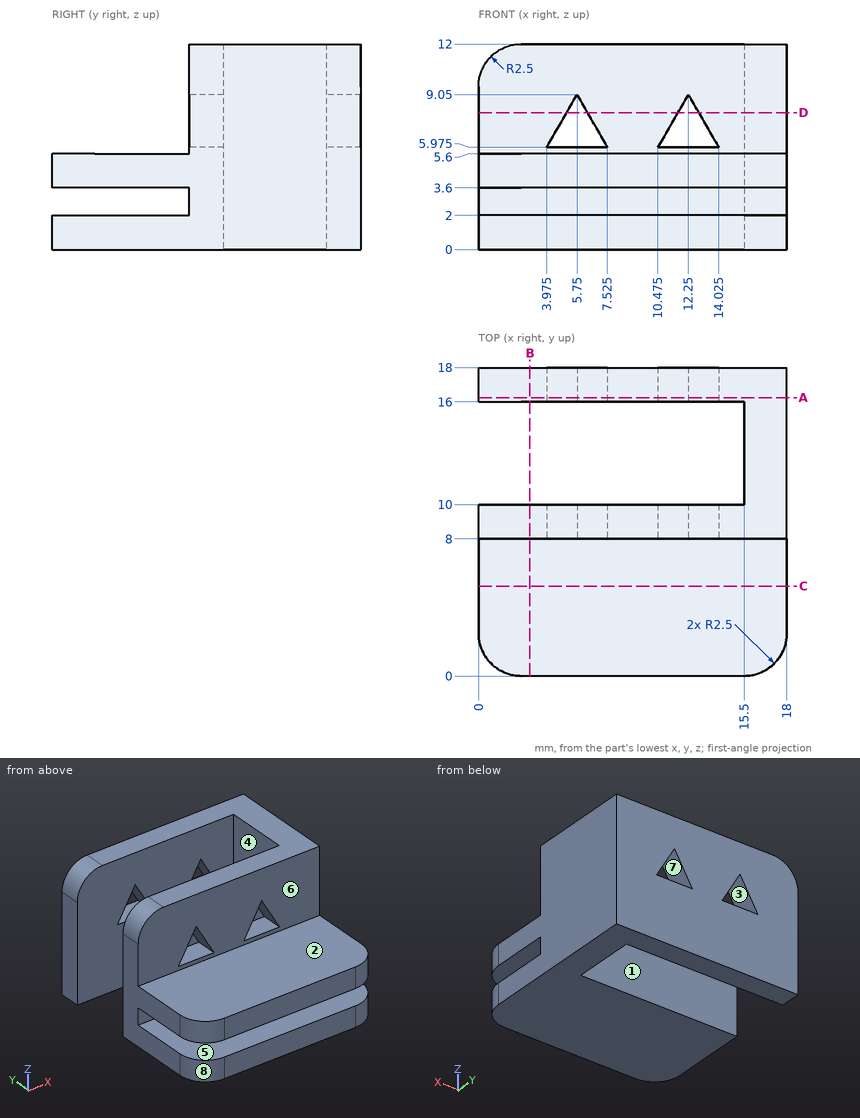
Geometry: see drawing. Coordinates: mm, zero at the bounding-box minimum. A direction names the side the tool comes from. Round coordinates to 2 decimals unless told otherwise and drop trailing zeros. Loops run counter-clockwise (first coordinate to the right, second up) from the corner with the lowest first, then second, coordinate; pieces in that order, holes last. Notation, with made-up numbers: (65, 25.25) -> (81, 25.25) arc R16 ccw to (81, 32.25) -> close; hole circle Ø10 at (-8.75, 89.5). An arc over 180 degrees is marked (long way). One line per question, with ' | ' between items. Start each with the question number.
1. Section C-C on y = 5.25. Output: boundary loops of the cut face in (x, z).
2. Set-up query: the marked faces 4, 5, 6, 7 and 8. Return all of +Z, -Z, +X, -X, +Y, -Y with unobstructed straight access to the full face (end or side cutting, diameter ignored); none if empty.
3. Contact query for flat-ended pins moving along their axis: pin 1 (5 mm diameter, centred on y = 13, z = 6.5, fed in from -X); pin 2 (2 mm diameter, centred on x = 8.5, y = 9.5, fed in from -Z); pin 3 (5 mm diameter, centred on x = 4, y = 3.5, fed in from +Z); pin 4 (3 mm diameter, centred on x = 12.5, z = 10.5, fed in from -Y). Output: stop coordinate, or through.
4. Mould query, pull axis Z, two halves, no side actions, for the marked faces 1, 2 and 3. Classes: pulls with the +Z half, pulls with the -Z half, needs draft (parallel to the pull), parting line crosses it, or undercut.
5. Section D-D on z = 8. Output: boundary loops of the cut face in (x, y).
6. Section A-A on y = 16.25. Count the separate pieces of the cut face and the enclosed holes in it, and give its area (3 significant figures).
7. Line query: line 1 along Y through (x, z) = (4.75, 2.5); line 2 along Z through (x, y) = (14, 2.75); line 3 along Y through (x, z) = (11.25, 3.75). Output: solid intervals per line, ascending. Write a range as [from, to].
8. Section B-B on x = 3. Output: boundary loops of the cut face in (y, z).
Returned:
1) outline: (0, 0) -> (18, 0) -> (18, 2) -> (0, 2) -> close; (0, 3.6) -> (18, 3.6) -> (18, 5.6) -> (0, 5.6) -> close
2) face 4: +Z, -Z, -X | face 5: +X, -X, -Y | face 6: +Z, +X, -X, -Y | face 7: +Y, -Y | face 8: +Z, -Z, -X, -Y
3) pin 1: stops at x = 15.5 | pin 2: stops at z = 0 | pin 3: stops at z = 5.6 | pin 4: stops at y = 8
4) face 1: needs draft | face 2: pulls with the +Z half | face 3: undercut
5) outline: (0, 8) -> (5.14, 8) -> (5.14, 10) -> (0, 10) -> close; (0, 16) -> (5.14, 16) -> (5.14, 18) -> (0, 18) -> close; (6.36, 8) -> (11.64, 8) -> (11.64, 10) -> (6.36, 10) -> close; (6.36, 16) -> (11.64, 16) -> (11.64, 18) -> (6.36, 18) -> close; (12.86, 8) -> (18, 8) -> (18, 18) -> (12.86, 18) -> (12.86, 16) -> (15.5, 16) -> (15.5, 10) -> (12.86, 10) -> close
6) separate pieces: 1 | enclosed holes: 2 | area: 204 mm2
7) line 1: y = [8, 10], [16, 18] | line 2: z = [0, 2], [3.6, 5.6] | line 3: y = [0, 10], [16, 18]
8) outline: (0, 0) -> (10, 0) -> (10, 12) -> (8, 12) -> (8, 5.6) -> (0, 5.6) -> (0, 3.6) -> (8, 3.6) -> (8, 2) -> (0, 2) -> close; (16, 0) -> (18, 0) -> (18, 12) -> (16, 12) -> close
